Here's how the part is built. I have some questions about the finished solid (model axes, mm). Face numbers are marked on the shaded views. A direction names the side the tool comes from. Coordinates: 2 decimals unless noted, no trailing zeros. Order: outer loops, then holes, each group sorted by start corner. A loop starts at its lowest first (then second) coordinate and runs counter-clockwise, first axis right, second up. Notation, with made-up numbers: (-28, 40) - (-5, 40) arc R20 cw to (-5, 75) - close; hole circle Ø2 at (33.25, -1.5). An arc over 180 degrees is marked (long way). Answer in a Markdown table with one row per item. Add a question column.
Item 1: Thinking about a two-plate mould opening in Y: for the marked faces 3, 4, 5 and 6, which applies, +Y half, -Y half, draft (parallel to the pull), parting line (faces both ways), or undercut?
Item 2: I want a section at C-C (x = -2.25). Please give me the cut outline in (y, z) (3 decimals), plus the area to 3 significant figures.
Item 3: I want a section at D-D (y = -6.25). Please give me the cut outline in (x, z) (3 decimals).
Item 4: I want a section at B-B (z = 2.05). Please give me the cut outline in (x, y).
Item 5: Will these pins go through, and if not, where does the flat tip stop? pin 1 Ø1 at (x, z) = (3, 2) entering from +Y; pin 2 Ø1 at (x, z) = (1.5, 0.5) entering from -Y; pin 3 Ø3 at (x, y) = (-0.04, 6.41) entering from -Z (3 decimals); pin 4 Ø1 at (x, y) = (-4, -4) entering from -Z.
Item 6: If I drill on line 1 along Z through (x, y) = (-1.25, 6) (3 decimals); line 2 along X through (y, z) = (0.5, 0.6); line 3 along X through (y, z) = (3, -0.05), over which ranges is the centre line in solid material (lowest first)? Write a range as from..to.
Item 7: On a 3-axis mill with a long thin cutter (end or side, diameter ignored), from which of +Z, -Z, +X, -X, +Y, -Y can I reach the whole of each face in a straight line? I mean the marked faces 1 and 2. Say none if no direction works.
Item 8: I want a section at A-A (z = -0.9). Please give me the cut outline in (x, y), plus the area to 3 significant figures.
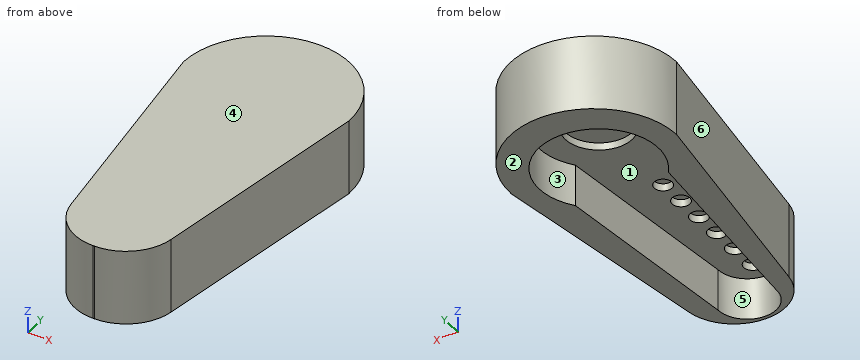
```python
from build123d import *

# Parameters (mm, degrees)
BOSS_EXTRUDE1_DEPTH = 0.45
SCALE2_SCALE        = 10
SKETCH4_R           = 0.5334
SKETCH4_R_2         = 2
CUT_EXTRUDE5_DEPTH  = 2.94
SKETCH4_3_R         = 0.5334
SKETCH4_3_R_2       = 2
CUT_EXTRUDE6_DEPTH  = 2.5
CUT_EXTRUDE7_DEPTH  = 4.5
FILLET5_R           = 3


with BuildPart() as part:
    # Sketch1 → Boss-Extrude1 (new body)
    with BuildSketch(Plane.XY):
        with BuildLine():
            Line((-0.136993219, -2.45), (0.163006781, -2.450375949))
            Line((0.163006781, -2.450375949), (0.499999859, -0.000375949))
            ThreePointArc((0.499999859, -0.000375949), (0.000187974, 0.499999965), (-0.5, 0))
            Line((-0.5, 0), (-0.136993219, -2.45))
        make_face()
    extrude(amount=BOSS_EXTRUDE1_DEPTH)


with BuildPart() as part_1:
    # Scale2: scaled about (0.004303075, -0.764400295, 0.225)
    add(part.part.scale(SCALE2_SCALE).moved(Location((-0.038727675, 6.879602655, -2.025))))

    # Sketch4 → Cut-Extrude5 (cut)
    with BuildSketch(Plane(origin=(0, 0, -2.025), x_dir=(-1, 0, 0), z_dir=(0, 0, -1))):
        with Locations((0.043782342, 0.298259193)):
            Circle(SKETCH4_R)
        with Locations((0.044722007, -1.403540547)):
            Circle(SKETCH4_R)
        with Locations((0.045661673, -3.105340288)):
            Circle(SKETCH4_R)
        with Locations((0.046601338, -4.807140028)):
            Circle(SKETCH4_R)
        with Locations((0.047541004, -6.508939769)):
            Circle(SKETCH4_R)
        with Locations((0.048480669, -8.21073951)):
            Circle(SKETCH4_R)
        with Locations((0.040405857, 6.413308261)):
            Circle(SKETCH4_R_2)
    extrude(amount=-CUT_EXTRUDE5_DEPTH, mode=Mode.SUBTRACT)

    # Sketch4<3> → Cut-Extrude6 (cut)
    with BuildSketch(Plane(origin=(0, 0, -2.025), x_dir=(-1, 0, 0), z_dir=(0, 0, -1))):
        with BuildLine():
            Line((1.794435881, -7.676375382), (2.854667965, 4.218872462))
            ThreePointArc((2.854667965, 4.218872462), (0.038435364, 9.982007717), (-2.771431177, 4.215765956))
            Line((-2.771431177, 4.215765956), (-1.698063587, -7.6783038))
            ThreePointArc((-1.698063587, -7.6783038), (0.049150356, -9.423589325), (1.794435881, -7.676375382))
        make_face()
        with Locations((0.043782342, 0.298259193)):
            Circle(SKETCH4_3_R, mode=Mode.SUBTRACT)
        with Locations((0.044722007, -1.403540547)):
            Circle(SKETCH4_3_R, mode=Mode.SUBTRACT)
        with Locations((0.045661673, -3.105340288)):
            Circle(SKETCH4_3_R, mode=Mode.SUBTRACT)
        with Locations((0.046601338, -4.807140028)):
            Circle(SKETCH4_3_R, mode=Mode.SUBTRACT)
        with Locations((0.047541004, -6.508939769)):
            Circle(SKETCH4_3_R, mode=Mode.SUBTRACT)
        with Locations((0.048480669, -8.21073951)):
            Circle(SKETCH4_3_R, mode=Mode.SUBTRACT)
        with Locations((0.040405857, 6.413308261)):
            Circle(SKETCH4_3_R_2, mode=Mode.SUBTRACT)
    extrude(amount=-CUT_EXTRUDE6_DEPTH, mode=Mode.SUBTRACT)

    # Sketch5 → Cut-Extrude7 (cut)
    with BuildSketch(Plane(origin=(0, 0, -2.025), x_dir=(-1, 0, 0), z_dir=(0, 0, -1))):
        Polygon((-2.691750397, -9.628866056), (2.593406399, -9.628866056), (1.408635162, -17.625106571), (-1.591364838, -17.628866056), align=None)
    extrude(amount=-CUT_EXTRUDE7_DEPTH, mode=Mode.SUBTRACT)

    # Fillet5
    fillet5_edges = [part_1.edges().sort_by_distance(p)[0] for p in [
        (-2.592733353, -9.628866056, 0.225),
        (2.691077951, -9.628866056, 0.225),
    ]]
    fillet(fillet5_edges, radius=FILLET5_R)


solid = part_1.part
```
Values follow:
| question | item | result |
|---|---|---|
| 1 | face 3 | undercut |
| 1 | face 4 | draft |
| 1 | face 5 | undercut |
| 1 | face 6 | -Y half |
| 2 | outline | (-8.618, -2.025) - (-2.565, -2.025) - (-2.565, 0.475) - (9.216, 0.475) - (9.216, -2.025) - (11.364, -2.025) - (11.364, 2.475) - (-8.618, 2.475) - close |
| 2 | area | 60.5 mm^2 |
| 3 | outline | (-3.093, -2.025) - (-1.922, -2.025) - (-1.922, 0.475) - (-0.514, 0.475) - (-0.514, 0.915) - (0.419, 0.915) - (0.419, 0.475) - (1.827, 0.475) - (1.827, -2.025) - (3.156, -2.025) - (3.156, 2.475) - (-3.093, 2.475) - close |
| 4 | outline | (-5.04, 6.88) - (-2.97, -7.07) arc R3 ccw to (0, -9.63) - (0.08, -9.63) arc R3 ccw to (3.05, -7.04) - (4.96, 6.88) arc R5 ccw to start |
| 5 | pin 1 | stops at y = 11.19 |
| 5 | pin 2 | stops at y = -9.48 |
| 5 | pin 3 | stops at z = 0.915 |
| 5 | pin 4 | passes through |
| 6 | line 1 | z = 0.915..2.475 |
| 6 | line 2 | x = -4.09..-0.54, 0.45..4.08 |
| 6 | line 3 | x = -4.46..-2.75, 2.66..4.43 |
| 7 | face 1 | -Z |
| 7 | face 2 | -Z, +X, -X, +Y, -Y |
| 8 | outline | (-5.04, 6.88) - (-2.97, -7.07) arc R3 ccw to (0, -9.63) - (0.08, -9.63) arc R3 ccw to (3.05, -7.04) - (4.96, 6.88) arc R5 ccw to start; hole (-2.85, 4.22) - (-1.79, -7.68) arc R1.75 ccw to (1.7, -7.68) - (2.77, 4.22) arc R3.57 ccw (long way) to start |
| 8 | area | 69.0 mm^2 |
